from build123d import *

# Parameters (mm, degrees)
F0_W      = 15
F0_H      = 15
F1_DEPTH  = 22.5
F2_R      = 12
F3_DEPTH  = 4
F4_D      = 3.3
F4_DEPTH  = 4
F4_TIP    = 0.9914200214
F6_D      = 3.3
F6_DEPTH  = 4
F6_TIP    = 0.9914200214
F7_R      = 6
F9_DEPTH  = 45
F11_D     = 3.3
F11_DEPTH = 4
F11_TIP   = 0.9914200214


# Not quite as in the source:
# - a pattern or mirror of a feature is missing from the dataset's text; its kind, count and spacing are read off the source's solid


with BuildPart() as f1:
    # F0 (on Top) → F1 (new body, symmetric)
    with BuildSketch(Plane.XY):
        with BuildLine():
            Line((-30.5995642671, 43.9848275573), (-45.610671266, 69.9848275573))
            Line((-45.610671266, 69.9848275573), (-49.0747728811, 67.9848275573))
            Line((-49.0747728811, 67.9848275573), (-12.9903810568, 5.4848275573))
            Line((-12.9903810568, 5.4848275573), (-26.5403215145, -2.3382342135))
            ThreePointArc((-26.5403215145, -2.3382342135), (-14.4977545891, -10.966881228), (0, -14.0151724427))
            ThreePointArc((0, -14.0151724427), (14.4977545891, -10.966881228), (26.5403215145, -2.3382342135))
            Line((26.5403215145, -2.3382342135), (12.9903810568, 5.4848275573))
            Line((12.9903810568, 5.4848275573), (49.0747728811, 67.9848275573))
            Line((49.0747728811, 67.9848275573), (45.610671266, 69.9848275573))
            Line((45.610671266, 69.9848275573), (30.5995642671, 43.9848275573))
            Line((30.5995642671, 43.9848275573), (28.2901631903, 39.9848275573))
            Line((28.2901631903, 39.9848275573), (12.0753804399, 11.9))
            Line((12.0753804399, 11.9), (0, 11.9))
            Line((0, 11.9), (-12.0753804399, 11.9))
            Line((-12.0753804399, 11.9), (-28.2901631903, 39.9848275573))
            Line((-28.2901631903, 39.9848275573), (-30.5995642671, 43.9848275573))
        make_face()
        Rectangle(F0_W, F0_H, mode=Mode.SUBTRACT)
        Polygon((0, 43.9848275573), (-30.5995642671, 43.9848275573), (-28.2901631903, 39.9848275573), (0, 39.9848275573), (28.2901631903, 39.9848275573), (30.5995642671, 43.9848275573), align=None)
    extrude(amount=F1_DEPTH, both=True)

    # F2 (on face) → F3 (cut, through all)
    with BuildSketch(Plane(origin=(0, 43.9848275573, 0), x_dir=(-1, 0, 0), z_dir=(0, 1, 0))):
        Circle(F2_R)
    extrude(amount=-F3_DEPTH, mode=Mode.SUBTRACT)

    # F4
    with Locations(Plane(origin=(0, 43.9848275573, 0), x_dir=(-1, 0, 0), z_dir=(0, 1, 0))):
        with Locations((15.5, 15.5), (15.5, -15.5), (-15.5, -15.5), (-15.5, 15.5)):
            Hole(F4_D / 2, depth=F4_DEPTH)
            with Locations((0, 0, -(F4_DEPTH + F4_TIP / 2))):  # 118° drill point
                Cone(0, F4_D / 2, F4_TIP, mode=Mode.SUBTRACT)

    # F6
    with Locations(Plane(origin=(-7.3677857926, -4.2537931107, 0), x_dir=(0.5, -0.8660254038, 0), z_dir=(-0.8660254038, -0.5, 0))):
        with Locations((-21.7451905284, -15), (-75.9139741771, -15), (-75.9139741771, 15), (-21.7451905284, 15)):
            f6 = Hole(F6_D / 2, depth=F6_DEPTH)
            with Locations((0, 0, -(F6_DEPTH + F6_TIP / 2))):  # 118° drill point
                Cone(0, F6_D / 2, F6_TIP, mode=Mode.SUBTRACT)

    # F6_copies: F6 across plane
    add(f6.mirror(Plane(origin=(0, 0, 0), x_dir=(0, 0, 1), z_dir=(1, 0, 0))), mode=Mode.SUBTRACT)

    # F7
    f7_edges = [f1.edges().sort_by_distance(p)[0] for p in [
        (-28.290163, 39.984828, 0),
        (-12.07538, 11.9, 0),
        (12.07538, 11.9, 0),
        (28.290163, 39.984828, 0),
        (-30.599564, 43.984828, 0),
        (30.599564, 43.984828, 0),
    ]]
    fillet(f7_edges, radius=F7_R)

    # F8 (on face) → F9 (cut, through all)
    with BuildSketch(Plane.XY.offset(22.5)):
        with BuildLine():
            Line((13.2199214619, -11.5), (-13.2199214619, -11.5))
            ThreePointArc((-13.2199214619, -11.5), (0, -14.0151724427), (13.2199214619, -11.5))
        make_face()
    extrude(amount=-F9_DEPTH, mode=Mode.SUBTRACT)

    # F11
    with Locations(Plane.XZ.offset(11.5)):
        with Locations((0, 15), (0, -15)):
            Hole(F11_D / 2, depth=F11_DEPTH)
            with Locations((0, 0, -(F11_DEPTH + F11_TIP / 2))):  # 118° drill point
                Cone(0, F11_D / 2, F11_TIP, mode=Mode.SUBTRACT)


solid = f1.part
Input: part model. Units: mm. Frame: model coordinates. A direction names the side the tool comes from. Coordinates: 2 decimals unless noted, no trailing zeros. Order: outer loops, then holes, each group sorted by start corner. A loop starts at its lowest first (then second) coordinate and runs counter-clockwise, first axis right, second up. Notation, with made-up numbers: M 16.25,12.5 L 25.25,12.5 A28 ccw 25.25,39.5 Z; hole C 47,85.5 d5. An arc over 180 degrees is marked long. One line per question, with ' | ' between items.
Item 1: Reachability of faces 4 (the flat face through (19.86, 1.52, 0.32)), 5 (the cylindrical face through (-13.926, 41.957, -15.004)), 6 (the flat face through (0, 11.9, 0)), 7 (the cylindrical face through (0.215, -9.472, -13.364)) from +Z, -Z, +X, -X, +Y, -Y: full face, straight path, thin tool, end or side. Return the list, or none.
Geometry results:
face 4: +Z, -Z, +X | face 5: +Y | face 6: +Z, -Z | face 7: -Y
Item 2: Draft query along Z for faces 1 (the cylindrical face through (-44.331, 63.824, -15.632)), 2 (the cylindrical face through (11.649, 12.726, 0.315)), 3 (the flat face through (0, 11, 22.5)). Return one class per face: released by +Z, released by -Z, zero draft, split by the parting line, or undercut.
Geometry results:
face 1: undercut | face 2: zero draft | face 3: released by +Z
Item 3: Section C-C (z = -18.5). Output: boundary loops of the cut face in (x, y).
Geometry results:
outline: M -49.07,67.98 L -12.99,5.48 L -26.54,-2.34 A36 ccw -13.22,-11.5 L 13.22,-11.5 A36 ccw 26.54,-2.34 L 12.99,5.48 L 49.07,67.98 L 45.61,69.98 L 32.33,46.98 A6 cw 27.14,43.98 L -27.14,43.98 A6 cw -32.33,46.98 L -45.61,69.98 Z; hole M -23.09,30.98 L -13.81,14.9 A6 ccw -8.61,11.9 L 8.61,11.9 A6 ccw 13.81,14.9 L 23.09,30.98 A6 ccw 17.9,39.98 L -17.9,39.98 A6 ccw Z; hole M -7.5,-7.5 L 7.5,-7.5 L 7.5,7.5 L -7.5,7.5 Z
Item 4: Section A-A (x = 0). Output: boundary loops of the cut face in (y, z), then the cut area to 3 significant figures.
Geometry results:
outline: M -11.5,-22.5 L -7.5,-22.5 L -7.5,-16.65 L -11.5,-16.65 Z; M -11.5,-13.35 L -7.5,-13.35 L -7.5,13.35 L -11.5,13.35 Z; M -11.5,16.65 L -7.5,16.65 L -7.5,22.5 L -11.5,22.5 Z; M 7.5,-22.5 L 11.9,-22.5 L 11.9,22.5 L 7.5,22.5 Z; M 39.98,-22.5 L 43.98,-22.5 L 43.98,-12 L 39.98,-12 Z; M 39.98,12 L 43.98,12 L 43.98,22.5 L 39.98,22.5 Z | area: 436 mm^2
Item 5: Section B-B (y = 22). Output: boundary loops of the cut face in (x, z), then the cut area to 3 significant figures.
Geometry results:
outline: M -22.53,-22.5 L -17.91,-22.5 L -17.91,22.5 L -22.53,22.5 Z; M 17.91,-22.5 L 22.53,-22.5 L 22.53,22.5 L 17.91,22.5 Z | area: 416 mm^2
Item 6: Pin query (flat end, axial travel): pin 1 (4.5 mm diameter, centred on y = 1, z = -10.5, fed in from -X); pin 2 (6 mm diameter, centred on x = 20.5, z = 15.5, fed in from +Y); pin 3 (1.5 mm diameter, centred on x = -17.5, y = 8.5, fed in from -Z); pin 4 (12 mm diameter, centred on x = -1.5, z = 2.5, fed in from +Y). Return the tip coordinate at first contact, or that it passes through.
Geometry results:
pin 1: stops at x = -24.66 | pin 2: stops at y = 43.98 | pin 3: passes through | pin 4: stops at y = 11.9
Item 7: Ray query, line 1 along Z through (x, y) = (15.5, 41.6); line 2 along Z through (x, y) = (0, -8.55); line 3 along Y through (x, z) = (-6, -18.5). Return the intervals inside material, ascending.
Geometry results:
line 1: z = -22.5 to -17.15, -13.85 to 13.85, 17.15 to 22.5 | line 2: z = -22.5 to -16.65, -13.35 to 13.35, 16.65 to 22.5 | line 3: y = -11.5 to -7.5, 7.5 to 11.9, 39.98 to 43.98
